Build history of the part. All positions in model axes, mm. A direction names the side the tool comes from. Round coordinates to 2 decimals unless told otherwise and drop trailing zeros. Order: outer loops, then holes, each group sorted by start corner. A loop starts at its lowest first (then second) coordinate and runs counter-clockwise, first axis right, second up. Notation, with made-up numbers: M -21,82 L -16,82 A22 cw -16,114 Z; hole C 23,53 d2. An arc over 180 degrees is marked long. Use CSV: the item, a comma, the result in double quotes.
from build123d import *

# Parameters (mm, degrees)
F0_R      = 3.9
F1_DEPTH  = 3
F3_R      = 1.95
F4_DEPTH  = 10
F7_R      = 1.4
F8_DEPTH  = 7
F5_R      = 0.95
F9_DEPTH  = 4.8
F10_DEPTH = 4.8


with BuildPart() as f1:
    # F0 (on Top) → F1 (new body)
    with BuildSketch(Plane.XY):
        Circle(F0_R)
    extrude(amount=F1_DEPTH)

    # F3 (on offset) → F4 (join)
    with BuildSketch(Plane.XY.offset(3)):
        Circle(F3_R)
    extrude(amount=F4_DEPTH)

    # F7 (on offset) → F8 (join)
    with BuildSketch(Plane.XY.offset(13)):
        Circle(F7_R)
    extrude(amount=F8_DEPTH)

    # F5 (on Front) → F9 (cut)
    with BuildSketch(Plane.XZ):
        with Locations((0, 11)):
            Circle(F5_R)
    extrude(amount=F9_DEPTH, mode=Mode.SUBTRACT)

    # F5 (on Front) → F10 (cut)
    with BuildSketch(Plane.XZ):
        with Locations((0, 11)):
            Circle(F5_R)
    extrude(amount=-F10_DEPTH, mode=Mode.SUBTRACT)


solid = f1.part
(1) Cut at C-C, the plane z = 7.5. Give the cut face in (x, y), and give its area (3 significant figures).
Answer block:
outline,"C 0,0 d3.9"
area,"11.9 mm²"
(2) Cut at A-A, the plane x = 0. Give the cut face in (y, z).
Answer block:
outline,"M -3.9,0 L 3.9,0 L 3.9,3 L 1.95,3 L 1.95,10.05 L -1.95,10.05 L -1.95,3 L -3.9,3 Z; M -1.95,11.95 L 1.95,11.95 L 1.95,13 L 1.4,13 L 1.4,20 L -1.4,20 L -1.4,13 L -1.95,13 Z"
(3) Wall check: line 1 (Z direction, x = 0, y = -0.6); line 2 (Z direction, x = -2.25, y = 3); line 3 (Z direction, x = -0.5, y = -1.5). Give the ranges that are in metal, low to high. Write a range as from..to.
Answer block:
line 1,"z = 0..10.05, 11.95..20"
line 2,"z = 0..3"
line 3,"z = 0..10.19, 11.81..13"
(4) Tool access for faces 4 (the face through (-2, -1, 3)), 5 (the face through (0, 0, 0)): list every direction of +Z, -Z, +X, -X, +Y, -Y with a clear straight run to the whole face (end or side of a thin tool).
Answer block:
face 4,"+Z"
face 5,"-Z, +X, -X, +Y, -Y"
(5) Drop flat-ended pins along their axis: pin 1 (1 mm diameter, centred on x = 1.5, z = 7.5, fed in from +Y); pin 2 (2 mm diameter, centred on x = 0, z = 11, fed in from -Y). Give the stop position or say it passes through.
Answer block:
pin 1,"stops at y = 1.67"
pin 2,"stops at y = -1.95"
(6) Cut at D-D, the plane z = 10.25. Give the cut face in (x, y), and give its area (3 significant figures).
Answer block:
outline,"M -0.58,-1.86 L -0.58,1.86 A1.95 ccw Z; M 0.58,-1.86 A1.95 ccw 0.58,1.86 Z"
area,"7.47 mm²"
(7) Two-plate mould, pull along X, no slides. Class faces 1 (the face through (0, 0, 20)), 2 (the face through (0.9, 0, 11.3)), 3 (the face through (-2.87, 2.64, 1.48)): released by +X, released by -X, zero draft, split by the parting line, or undercut.
Answer block:
face 1,"zero draft"
face 2,"undercut"
face 3,"split by the parting line"
(8) Cut at B-B, the plane y = 0. Give the cut face in (x, z), and give its area (3 significant figures).
Answer block:
outline,"M -3.9,0 L 3.9,0 L 3.9,3 L 1.95,3 L 1.95,13 L 1.4,13 L 1.4,20 L -1.4,20 L -1.4,13 L -1.95,13 L -1.95,3 L -3.9,3 Z; hole C 0,11 d1.9"
area,"79.2 mm²"
